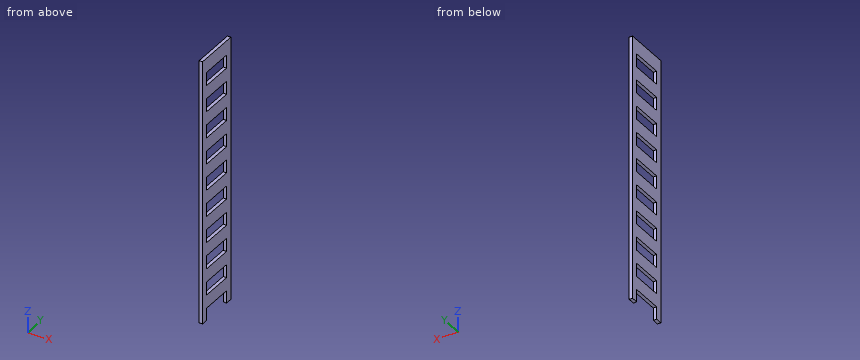
from build123d import *

# Parameters (mm, degrees)
SKETCH1_W           = 60
SKETCH1_H           = 140
BOSS_EXTRUDE1_DEPTH = 15


with BuildPart() as part:
    # Sketch1 → Boss-Extrude1 (new body)
    with BuildSketch(Plane(origin=(0, 0, 0), x_dir=(0, 0, -1), z_dir=(1, 0, 0))):
        Polygon((-600.7, 0), (600.7, 0), (600.7, 30), (544.3, 30), (544.3, 170), (600.7, 170), (600.7, 200), (-600.7, 200), align=None)
        with Locations((-505.7, 100)):
            Rectangle(SKETCH1_W, SKETCH1_H, mode=Mode.SUBTRACT)
        with Locations((-385.7, 100)):
            Rectangle(SKETCH1_W, SKETCH1_H, mode=Mode.SUBTRACT)
        with Locations((-265.7, 100)):
            Rectangle(SKETCH1_W, SKETCH1_H, mode=Mode.SUBTRACT)
        with Locations((-145.7, 100)):
            Rectangle(SKETCH1_W, SKETCH1_H, mode=Mode.SUBTRACT)
        with Locations((-25.7, 100)):
            Rectangle(SKETCH1_W, SKETCH1_H, mode=Mode.SUBTRACT)
        with Locations((94.3, 100)):
            Rectangle(SKETCH1_W, SKETCH1_H, mode=Mode.SUBTRACT)
        with Locations((214.3, 100)):
            Rectangle(SKETCH1_W, SKETCH1_H, mode=Mode.SUBTRACT)
        with Locations((334.3, 100)):
            Rectangle(SKETCH1_W, SKETCH1_H, mode=Mode.SUBTRACT)
        with Locations((454.3, 100)):
            Rectangle(SKETCH1_W, SKETCH1_H, mode=Mode.SUBTRACT)
    extrude(amount=BOSS_EXTRUDE1_DEPTH)


solid = part.part
Here's how the part is built. I have some questions about the finished solid (model axes, mm). Round coordinates to 2 decimals unless told otherwise and drop trailing zeros. Order: outer loops, then holes, each group sorted by start corner. A loop starts at its lowest first (then second) coordinate and runs counter-clockwise, first axis right, second up. Notation, with made-up numbers: M -39.75,66.25 L -18.75,66.25 A24 cw -18.75,80.25 Z; hole C 11.5,68 d5. An arc over 180 degrees is marked long. Return JSON: item names as keys, results as strings. Group by question number.
1. If we section it at B-B on y = 160: State how many separate pieces and enclosed holes the cut face has, then the cut area to 4 significant figures.
2. Please list where this line runs through material, in increasing order: probe 1 along Y at (x, z) = (9.25, -348.5).
3. I'm going to push a flat-ended pin straight in: pin 1 Ø2 at (x, y) = (12, 117.5) entering from -Z. Where does the tip first touch, or does it pass through?
4. If we section it at A-A on z = -338: List the corners of the cut face in (x, y) for me, then the cut area to 3 significant figures.
Reply:
{
 "1": {"separate pieces": "10", "enclosed holes": "0", "area": "9,075 mm^2"},
 "2": {"probe 1": "0 to 30, 170 to 200"},
 "3": {"pin 1": "z = -544.3"},
 "4": {"outline": "M 0,0 L 15,0 L 15,30 L 0,30 Z; M 0,170 L 15,170 L 15,200 L 0,200 Z", "area": "900 mm^2"}
}
